Work out the finished part from the listing and answer in its coordinate system (mm). A direction names the side the tool comes from. Coordinates: 2 decimals unless noted, no trailing zeros. Write each loop counter-clockwise with the first axis right and the second up, starting at its lowest first coordinate (ties: lowest second). Pieces come first, ordered by that corner, then holes. Notation, with made-up numbers: (-0.5, -17.75) - (20.5, -17.75) arc R23 ccw to (20.5, 15.25) - close; hole circle Ø6 at (85, 39.5). An arc over 180 degrees is marked (long way). Use a Markdown table: item, result. Add a question column.
(1) The part is cut by section A-A, the plane x = 137. Give the vertices of the cut face in (y, z).
(2) For a pull along Y with two mould halves and no side action, classify faces 1 (the face through (101, 0, 222)), 2 (the face through (0.28, 5.32, 221.85)), 3 (the face through (100.766, 4.536, 445.271)), 4 (the face through (162.821, 23, 224)) as released by +Y, released by -Y, zero draft, split by the parting line, or undercut.
(3) Given pin 1 Ø4 at (y, z) = (-4, 137) entering from -X; pin 2 Ø6.5 at (x, y) = (54.5, 13) entering from -Z; pin 3 Ø3 at (x, z) = (114.5, 244) entering from -Y; pin 4 Ø3 at (x, y) = (29, 8) entering from +Z, each flat-ended and moving along its own axis, determine where each tip first touches the part or whether it passes through.
(4) Find the intervals of material crossed by line 1 (Z direction, x = 9, y = 15.5); line 2 (Y direction, x = 141.5, z = 94); line 3 (Z direction, x = 75, y = 12), in increasing order. Write a range as from..to.
(5) The part is cut by section B-B, the plane z = 298. Give the vertices of the cut face in (x, y).
(6) A tool of negligible diameter and unlimited length cuts with its end or side. For faces 5 (the face through (81, 16, 449)), 6 (the face through (89, 22.2, 222)), 7 (the face through (100.77, 3.82, 4.03)), from which of +Z, -Z, +X, -X, +Y, -Y can it reach the whole face along a straight path? Write none if from no direction.
from build123d import *

# Parameters (mm, degrees)
BOSS_EXTRUDE1_DEPTH = 450
FILLET1_R           = 13.4
BOSS_EXTRUDE2_DEPTH = 450
FILLET2_R           = 13.4
CUT_EXTRUDE1_DEPTH  = 451.0000001
SHELL1_T            = -1
BOSS_EXTRUDE3_DEPTH = 450
CUT_EXTRUDE2_DEPTH  = 13.698698186


with BuildPart() as part:
    # Sketch2 → Boss-Extrude1 (new body)
    with BuildSketch(Plane.XY):
        Polygon((0, 0), (162.820860479, 0), (162.820860479, 23.2), (1.215860479, 23.2), align=None)
    extrude(amount=BOSS_EXTRUDE1_DEPTH)

    # Fillet1
    fillet1_edges = [part.edges().sort_by_distance(p)[0] for p in [
        (1.215860479, 23.2, 225),
    ]]
    fillet(fillet1_edges, radius=FILLET1_R)

    # Sketch4 → Boss-Extrude2 (add, through all)
    with BuildSketch(Plane.XY.offset(450)):
        with BuildLine():
            Line((24.166834741, -1.266530141), (23.567700201, -12.698698186))
            ThreePointArc((23.567700201, -12.698698186), (27.725384653, -3.679983428), (36.949335967, 0))
            Line((36.949335967, 0), (0, 0))
            Line((0, 0), (9.586843534, -0.50242518))
            Line((9.586843534, -0.50242518), (9.22049184, -7.492831923))
            Line((9.22049184, -7.492831923), (14.213639514, -7.754511704))
            Line((14.213639514, -7.754511704), (14.579991207, -0.764104961))
            Line((14.579991207, -0.764104961), (24.166834741, -1.266530141))
        make_face()
    extrude(amount=-BOSS_EXTRUDE2_DEPTH)

    # Fillet2
    fillet2_edges = [part.edges().sort_by_distance(p)[0] for p in [
        (27.725384653, -3.679983428, 0),
        (27.725384653, -3.679983428, 450),
        (99.885098223, 0, 450),
        (99.885098223, 0, 0),
    ]]
    fillet(fillet2_edges, radius=FILLET2_R)

    # Sketch5 → Cut-Extrude1 (cut, through all)
    with BuildSketch(Plane.XY):
        with BuildLine():
            Line((24.166834741, -1.266530141), (23.567700201, -12.698698186))
            ThreePointArc((23.567700201, -12.698698186), (27.725384653, -3.679983428), (36.949335967, 0))
            Line((36.949335967, 0), (0, 0))
            Line((0, 0), (9.586843534, -0.50242518))
            Line((9.586843534, -0.50242518), (9.22049184, -7.492831923))
            Line((9.22049184, -7.492831923), (14.213639514, -7.754511704))
            Line((14.213639514, -7.754511704), (14.579991207, -0.764104961))
            Line((14.579991207, -0.764104961), (24.166834741, -1.266530141))
        make_face()
    extrude(amount=CUT_EXTRUDE1_DEPTH, mode=Mode.SUBTRACT)

    # Shell1
    shell1_openings = [part.faces().sort_by_distance(p)[0] for p in [
        (162.820860479, 11.274923044, 225),
    ]]
    offset(amount=SHELL1_T, openings=shell1_openings)

    # Sketch6 → Boss-Extrude3 (add)
    with BuildSketch(Plane.XY):
        with BuildLine():
            Line((24.166834741, -1.266530141), (23.567700201, -12.698698186))
            ThreePointArc((23.567700201, -12.698698186), (27.725384653, -3.679983428), (36.949335967, 0))
            Line((36.949335967, 0), (0, 0))
            Line((0, 0), (9.586843534, -0.50242518))
            Line((9.586843534, -0.50242518), (9.22049184, -7.492831923))
            Line((9.22049184, -7.492831923), (14.213639514, -7.754511704))
            Line((14.213639514, -7.754511704), (14.579991207, -0.764104961))
            Line((14.579991207, -0.764104961), (24.166834741, -1.266530141))
        make_face()
    extrude(amount=BOSS_EXTRUDE3_DEPTH)

    # Sketch7 → Cut-Extrude2 (cut, through all)
    with BuildSketch(Plane.XZ):
        with BuildLine():
            Line((13.739855146, 450), (36.949335967, 450))
            Line((36.949335967, 450), (36.949335967, 436.6))
            add(Edge.make_bspline(
                [(13.739855146, 450), (14.897031698, 450), (16.037346218, 449.888583323), (17.726143963, 449.5782461), (18.285436938, 449.450751492), (19.397111441, 449.150094553), (19.951343846, 448.976153087), (22.667401959, 448.011694289), (24.688899416, 446.937288096), (27.088419743, 445.339458648), (27.560915156, 445.007570641), (28.487586558, 444.326213533), (28.942650844, 443.976156414), (30.286745236, 442.902062513), (31.15469064, 442.154118787), (32.853186658, 440.615831161), (33.683710559, 439.825456971), (35.32594722, 438.223379533), (36.139219776, 437.410115889), (36.949335967, 436.6)],
                knots=[0, 0, 0, 0, 0.125, 0.125, 0.1875, 0.1875, 0.25, 0.25, 0.5, 0.5, 0.5625, 0.5625, 0.625, 0.625, 0.75, 0.75, 0.875, 0.875, 1, 1, 1, 1], degree=3))
        make_face()
        with BuildLine():
            Line((36.949335967, 13.4), (36.949335967, 0))
            Line((36.949335967, 0), (13.739855146, 0))
            add(Edge.make_bspline(
                [(36.949335967, 13.4), (36.139219776, 12.589884111), (35.32594722, 11.776620467), (33.683710559, 10.174543029), (32.853186658, 9.384168839), (31.15469064, 7.845881213), (30.286745236, 7.097937487), (28.942650844, 6.023843586), (28.487586558, 5.673786467), (27.560915156, 4.992429359), (27.088419743, 4.660541352), (24.688899416, 3.062711904), (22.667401959, 1.988305711), (19.951343846, 1.023846913), (19.397111441, 0.849905447), (18.285436938, 0.549248508), (17.726143963, 0.4217539), (16.037346218, 0.111416677), (14.897031698, 0), (13.739855146, 0)],
                knots=[0, 0, 0, 0, 0.125, 0.125, 0.25, 0.25, 0.375, 0.375, 0.4375, 0.4375, 0.5, 0.5, 0.75, 0.75, 0.8125, 0.8125, 0.875, 0.875, 1, 1, 1, 1], degree=3))
        make_face()
    extrude(amount=CUT_EXTRUDE2_DEPTH, mode=Mode.SUBTRACT)


solid = part.part
Model answer:
| question | item | result |
|---|---|---|
| 1 | outline | (0, 13.4) arc R13.4 ccw to (13.4, 0) - (23.2, 0) - (23.2, 450) - (13.4, 450) arc R13.4 ccw to (0, 436.6) - close; hole (1, 13.4) arc R12.4 ccw to (13.4, 1) - (22.2, 1) - (22.2, 449) - (13.4, 449) arc R12.4 ccw to (1, 436.6) - close |
| 2 | face 1 | released by -Y |
| 2 | face 2 | released by +Y |
| 2 | face 3 | undercut |
| 2 | face 4 | zero draft |
| 3 | pin 1 | x = 9.3 |
| 3 | pin 2 | z = 0 |
| 3 | pin 3 | y = 0 |
| 3 | pin 4 | z = 449.77 |
| 4 | line 1 | 0..1, 449..450 |
| 4 | line 2 | 0..1, 22.2..23.2 |
| 4 | line 3 | 0.07..1.08, 448.92..449.93 |
| 5 | outline | (0, 0) - (9.59, -0.5) - (9.22, -7.49) - (14.21, -7.75) - (14.58, -0.76) - (24.17, -1.27) - (23.57, -12.7) arc R13.4 cw to (36.95, 0) - (162.82, 0) - (162.82, 1) - (1.05, 1) - (1.55, 10.45) arc R12.4 cw to (13.93, 22.2) - (162.82, 22.2) - (162.82, 23.2) - (13.93, 23.2) arc R13.4 ccw to (0.55, 10.5) - close |
| 6 | face 5 | none |
| 6 | face 6 | +X |
| 6 | face 7 | -Z, +X, -Y |
